```python
from build123d import *

# Parameters (mm, degrees)
SKETCH1_R           = 50
BOSS_EXTRUDE1_DEPTH = 24
FILLET1_R           = 12
SKETCH2_R           = 11
CUT_EXTRUDE1_DEPTH  = 6.5
CUT_EXTRUDE2_START  = -6.5
SKETCH3_R           = 11
CUT_EXTRUDE2_DEPTH  = 6.5
SKETCH4_R           = 9
CUT_EXTRUDE3_DEPTH  = 73.844011422


with BuildPart() as part:
    # Sketch1 → Boss-Extrude1 (new body)
    with BuildSketch(Plane(origin=(0, 0, 0), x_dir=(1, 0, 0), z_dir=(0, 1, 0))):
        with Locations(Location((0, 0, 0), (0, 0, 270))):
            Circle(SKETCH1_R)
    extrude(amount=BOSS_EXTRUDE1_DEPTH)

    # Fillet1
    fillet1_edges = [part.edges().sort_by_distance(p)[0] for p in [
        (0, 0, -50),
        (0, 24, -50),
    ]]
    fillet(fillet1_edges, radius=FILLET1_R - 0.0001)  # a hair under: the kernel refuses the full size

    # Sketch2 → Cut-Extrude1 (cut)
    with BuildSketch(Plane(origin=(0, 24, 0), x_dir=(1, 0, 0), z_dir=(0, 1, 0))):
        with Locations(Location((0, 0, 0), (0, 0, 270))):
            Circle(SKETCH2_R)
    extrude(amount=-CUT_EXTRUDE1_DEPTH, mode=Mode.SUBTRACT)

    # Sketch3 → Cut-Extrude2 (cut)
    with BuildSketch(Plane.XZ.offset(CUT_EXTRUDE2_START)):
        with Locations(Location((0, 0, 0), (0, 0, 90))):
            Circle(SKETCH3_R)
    extrude(amount=CUT_EXTRUDE2_DEPTH, mode=Mode.SUBTRACT)

    # Sketch4 → Cut-Extrude3 (cut, through all)
    with BuildSketch(Plane.XZ.offset(-6.5)):
        with Locations(Location((0, 0, 0), (0, 0, 270))):
            Circle(SKETCH4_R)
    extrude(amount=-CUT_EXTRUDE3_DEPTH, mode=Mode.SUBTRACT)


solid = part.part
```
The listing builds one solid part. Answer for the finished solid, in the listing's coordinates (mm). A direction names the side the tool comes from. Give positions to 0.01 mm unless a question says otherwise; leave off trailing zeros. Write each loop counter-clockwise with the first axis right and the second up, starting at its lowest first coordinate (ties: lowest second). Pieces come first, ordered by that corner, then holes. Notation, with made-up numbers: (76.25, 36.5) -> (89.25, 36.5) arc R16 cw to (89.25, 57.5) -> close; hole circle Ø2 at (-33, 24.25). An arc over 180 degrees is marked (long way). Write item = value, one per line. Start each with the question number.
1) The part is cut by section D-D, the plane y = 8.5. Determine the outline of the cut face in (x, z).
2) Which of the six approach directions +Z, -Z, +X, -X, +Y, -Y give full straight-line access (tool end or side, diameter ignored) to faces 3 (the face through (-8, 0, 8)), 4 (the face through (-10.74, 20.8, -2.38)), 5 (the face through (10.74, 3.3, -2.38))?
3) Straight lines are drawn through the part: line 1 along X through (y, z) = (11.5, 0); line 2 along X through (y, z) = (3, -4); line 3 along Y through (x, z) = (37, -10). For each, find the intervals that lie inside material, in ascending order.
4) Each of these flat-tipped pins is pushed along its axis until it touches: pin 1 (4 mm diameter, centred on x = 24, z = 33.5, fed in from -Y); pin 2 (1.5 mm diameter, centred on y = 9.5, z = 2, fed in from -X); pin 3 (5 mm diameter, centred on x = -39.5, z = -22.5, fed in from -Y); pin 4 (6.5 mm diameter, centred on x = -3, z = -3, fed in from -Y). Where does it stop, or does it pass through?
5) The part is cut by section C-C, the plane y = 20.25. Determine the outline of the cut face in (x, z), and give its area (3 significant figures).
6) Determine the mould class of faces 1 (the face through (-8, 24, 8)), 2 (the face through (-9, 17.5, 2)) for opening direction X: +X half, -X half, draft (parallel to the pull), parting line (faces both ways), or undercut.
Solutions:
q1.outline = circle Ø98.96 at (0, 0); hole circle Ø18 at (0, 0)
q2.face_3 = +Z, -Z, +X, -X, -Y
q2.face_4 = +Y
q2.face_5 = -Y
q3.line_1 = -49.99 to -9, 9 to 49.99
q3.line_2 = -45.76 to -10.25, 10.25 to 45.76
q3.line_3 = 0 to 24
q4.pin_1 = 0.06
q4.pin_2 = -49.84
q4.pin_3 = 1.07
q4.pin_4 = through
q5.outline = circle Ø93.43 at (0, 0); hole circle Ø22 at (0, 0)
q5.area = 6,480 mm²
q6.face_1 = draft
q6.face_2 = undercut
